```python
from build123d import *

# Parameters (mm, degrees)
F0_W          = 40
F0_H          = 20
F1_DEPTH      = 120
F1_DEPTH_BACK = 100
F2_R          = 15
F3_DEPTH      = 15
F4_SIZE       = 5


with BuildPart() as f1:
    # F0 (on Top) → F1 (new body, two sides)
    with BuildSketch(Plane.XY) as f1_sk:
        with Locations((0, 10)):
            Rectangle(F0_W, F0_H)
    extrude(amount=F1_DEPTH)
    extrude(f1_sk.sketch, amount=-F1_DEPTH_BACK)

    # F2 (on face) → F3 (join)
    with BuildSketch(Plane.XZ):
        with Locations((0, 80)):
            Circle(F2_R)
    extrude(amount=F3_DEPTH)

    # F4
    f4_edges = [f1.edges().sort_by_distance(p)[0] for p in [
        (0, 0, 120),
        (20, 10, 120),
        (0, 20, 120),
        (-20, 10, 120),
    ]]
    chamfer(f4_edges, length=F4_SIZE)


solid = f1.part
```
Geometry check sheet. Reference: the model listing, model coordinates, mm. A direction names the side the tool comes from. Coordinates: 2 decimals unless noted, no trailing zeros. Loops run counter-clockwise (first coordinate to the right, second up) from the corner with the lowest first, then second, coordinate; pieces in that order, holes last.
Item 1: Sectioned sample at A-A, the plane x = 0. Record the boundary of the cut face in (y, z).
Item 2: Sectioned sample at C-C, the plane y = -6.5. Record the boundary of the cut face in (x, z).
Item 3: Sectioned sample at B-B, the plane z = 80. Record the boundary of the cut face in (x, y).
Item 4: Access from +Z, -Z, +X, -X, +Y, -Y to the whole of each face (thin tool, end or side, straight path). Record for faces 1 (the face through (-3.252, -7.395, 65.357)), 2 (the face through (0, -15, 80)).
Item 5: Go/stop test with a flat-tipped pin: pin 1 Ø2 at (x, z) = (7, -24) entering from -Y. Record where the tip stops, or that it passes through.
Item 6: Sectioned sample at D-D, the plane z = -79. Record the boundary of the cut face in (x, y).
Item 7: Thickness scan on line 1 (Y direction, x = -5.5, z = -86.5); line 2 (Z direction, x = 0, y = -3.5); line 3 (Z direction, x = 5.5, y = 4). Record the ranges inside material, lowest first.
Check result:
1. outline: (-15, 65) - (0, 65) - (0, -100) - (20, -100) - (20, 115) - (15, 120) - (5, 120) - (0, 115) - (0, 95) - (-15, 95) - close
2. outline: circle Ø30 at (0, 80)
3. outline: (-20, 0) - (-15, 0) - (-15, -15) - (15, -15) - (15, 0) - (20, 0) - (20, 20) - (-20, 20) - close
4. face 1: -Y
4. face 2: +Z, -Z, +X, -X, -Y
5. pin 1: stops at y = 0
6. outline: (-20, 0) - (20, 0) - (20, 20) - (-20, 20) - close
7. line 1: y = 0 to 20
7. line 2: z = 65 to 95
7. line 3: z = -100 to 119
